from build123d import *

# Parameters (mm, degrees)
F1_DEPTH = 57.15
F2_R     = 1.778
F3_DEPTH = 19.051
F4_R     = 5.08
F5_SIZE  = 8.89


with BuildPart() as f1:
    # F0 (on Front) → F1 (new body)
    with BuildSketch(Plane.XZ):
        Polygon((0, 16.51), (0, 0), (19.05, 0), (19.05, 16.51), (16.51, 16.51), (16.51, 2.54), (2.54, 2.54), (2.54, 16.51), align=None)
    extrude(amount=F1_DEPTH)

    # F2 (on face) → F3 (cut, through all)
    with BuildSketch(Plane(origin=(0, 0, 0), x_dir=(0, -1, 0), z_dir=(-1, 0, 0))):
        with Locations((6.604, 9.906)):
            Circle(F2_R)
    extrude(amount=-F3_DEPTH, mode=Mode.SUBTRACT)

    # F4
    f4_edges = [f1.edges().sort_by_distance(p)[0] for p in [
        (17.78, 0, 16.51),
        (1.27, 0, 16.51),
    ]]
    fillet(f4_edges, radius=F4_R)

    # F5
    f5_edges = [f1.edges().sort_by_distance(p)[0] for p in [
        (1.27, -57.15, 16.51),
        (17.78, -57.15, 16.51),
    ]]
    chamfer(f5_edges, length=F5_SIZE)


solid = f1.part
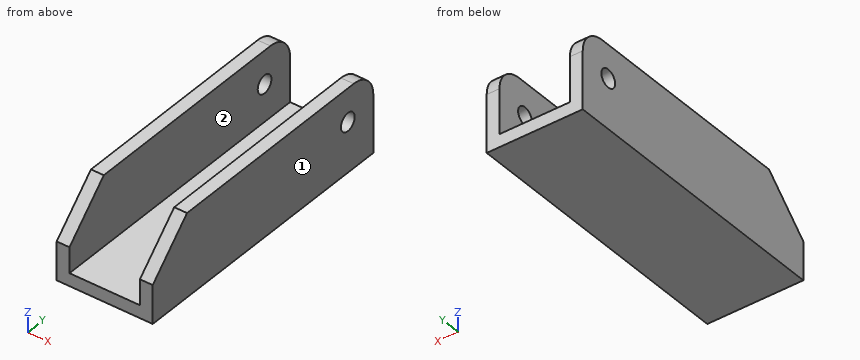
Geometry check sheet. Reference: the model listing, model coordinates, mm. Face numbers are marked on the shaded views. A direction names the side the tool comes from. Coordinates: 2 decimals unless noted, no trailing zeros. Loops run counter-clockwise (first coordinate to the right, second up) from the corner with the lowest first, then second, coordinate; pieces in that order, holes last. Notation, with made-up numbers: (-32, -3) - (-1, -3) arc R12 ccw to (-1, 7) - close; hole circle Ø1 at (75.5, 56). An arc over 180 degrees is marked (long way). Use one line per item in the form item = value. Start each with the question number.
Item 1: Section check C-C, the plane x = 2. Enter the section's corners in (y, z).
Item 2: Tool access check on the marked faces 1 and 2. Record the directions out of +Z, -Z, +X, -X, +Y, -Y that give a thin tool (end or side, any length) a straight path to the whole face; none if there is none.
Item 3: Gauge pin test, flat end, axial feed: pin 1 (8 mm diameter, centred on x = 8, y = -17, fed in from +Z). Record the tip position at first contact, or that the pin passes through.
Item 4: Thickness scan on probe 1 along X at (y, z) = (-18, 10.5); probe 2 along Z at (x, y) = (10, -30); probe 3 along Z at (x, y) = (16.75, -8). Record the ranges inside material, lowest first.
Item 5: Section check B-B, the plane y = -42. Enter the section's corners in (x, z).
Item 6: Section check A-A, the plane z = 5. Enter the section's corners in (x, y), and give its area (3 significant figures).
Item 7: Section check D-D, the plane z = 10.5. Enter the section's corners in (x, y).
Computed:
q1.outline = (-57.15, 0) - (0, 0) - (0, 11.43) arc R5.08 ccw to (-5.08, 16.51) - (-48.26, 16.51) - (-57.15, 7.62) - close; hole circle Ø3.56 at (-6.6, 9.91)
q2.face_1 = +Z, -Z, +X, +Y, -Y
q2.face_2 = +Z, +Y, -Y
q3.pin_1 = 2.54
q4.probe_1 = 0 to 2.54, 16.51 to 19.05
q4.probe_2 = 0 to 2.54
q4.probe_3 = 0 to 8.8, 11.01 to 16.51
q5.outline = (0, 0) - (19.05, 0) - (19.05, 16.51) - (16.51, 16.51) - (16.51, 2.54) - (2.54, 2.54) - (2.54, 16.51) - (0, 16.51) - close
q6.outline = (0, -57.15) - (2.54, -57.15) - (2.54, 0) - (0, 0) - close; (16.51, -57.15) - (19.05, -57.15) - (19.05, 0) - (16.51, 0) - close
q6.area = 290 mm2
q7.outline = (0, -54.27) - (2.54, -54.27) - (2.54, -8.28) - (0, -8.28) - close; (0, -4.93) - (2.54, -4.93) - (2.54, 0) - (0, 0) - close; (16.51, -54.27) - (19.05, -54.27) - (19.05, -8.28) - (16.51, -8.28) - close; (16.51, -4.93) - (19.05, -4.93) - (19.05, 0) - (16.51, 0) - close
